Could you check a few things on this model? Use its own coordinates, in mm. Face numbers are marked on the shaded views. A direction names the side the tool comes from. Give positions to 0.01 mm unless a question says otherwise; leave off trailing zeros. Loops run counter-clockwise (first coordinate to the right, second up) from the corner with the lowest first, then second, coordinate; pieces in that order, holes last. Notation, with made-up numbers: M -1.75,-27.5 L 37.25,-27.5 A14 ccw 37.25,-18.5 Z; hole C 13.5,-6 d8. An arc over 180 degrees is marked long. Write each question's results on one line, items separated by ' | '. Start each with the question number.
from build123d import *

# Parameters (mm, degrees)
F0_W     = 101.5878766775
F0_H     = 24.442197755
F1_DEPTH = 20
F3_DEPTH = 25
F5_DEPTH = 25


with BuildPart() as f1:
    # F0 (on Top) → F1 (new body)
    with BuildSketch(Plane.XY):
        with Locations((0.3819093108, 12.2210988775)):
            Rectangle(F0_W, F0_H)
    extrude(amount=F1_DEPTH)

    # F2 (on face) → F3 (cut)
    with BuildSketch(Plane.XY.offset(20)):
        with BuildLine():
            ThreePointArc((-50.4120290279, 16.5795714258), (-49.5897410565, 20.6289075462), (-47.9984842241, 24.442197755))
            Line((-47.9984842241, 24.442197755), (-50.4120290279, 24.442197755))
            Line((-50.4120290279, 24.442197755), (-50.4120290279, 16.5795714258))
        make_face()
        with BuildLine():
            ThreePointArc((-47.9984842241, 0), (-49.6724374157, 4.6588518495), (-50.4120290279, 9.5537496105))
            Line((-50.4120290279, 9.5537496105), (-50.4120290279, 0))
            Line((-50.4120290279, 0), (-47.9984842241, 0))
        make_face()
        with BuildLine():
            Line((51.1758476496, 24.442197755), (47.9984171689, 24.442197755))
            ThreePointArc((47.9984171689, 24.442197755), (50.12222675, 20.4607446272), (51.1758476496, 16.0729867548))
            Line((51.1758476496, 16.0729867548), (51.1758476496, 24.442197755))
        make_face()
        with BuildLine():
            Line((51.1758476496, 0), (51.1758476496, 12.2210988775))
            ThreePointArc((51.1758476496, 12.2210988775), (50.425198292, 5.9349952856), (48.2219271362, 0))
            Line((48.2219271362, 0), (51.1758476496, 0))
        make_face()
    extrude(amount=-F3_DEPTH, mode=Mode.SUBTRACT)

    # F4 (on face) → F5 (cut)
    with BuildSketch(Plane.XY.offset(20)):
        with BuildLine():
            ThreePointArc((-47.9984842241, 24.442197755), (-45.641486399, 24.1705843884), (-43.4080474079, 23.3699828386))
            Line((-43.4080474079, 23.3699828386), (44.5075258613, 23.3699828386))
            ThreePointArc((44.5075258613, 23.3699828386), (46.1724950081, 24.1681037554), (47.9984171689, 24.442197755))
            Line((47.9984171689, 24.442197755), (-47.9984842241, 24.442197755))
        make_face()
    extrude(amount=-F5_DEPTH, mode=Mode.SUBTRACT)


solid = f1.part
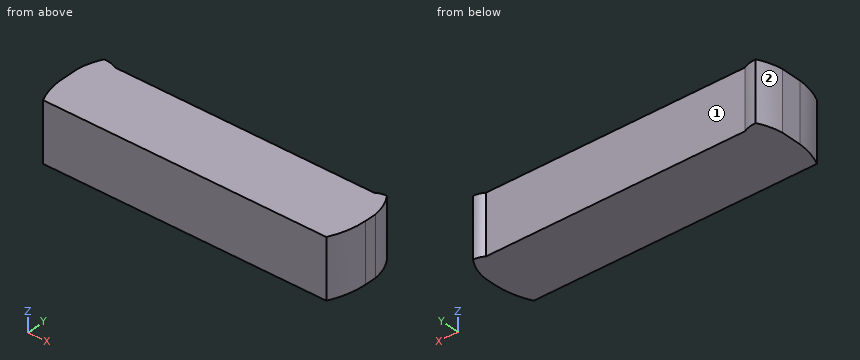
1) If we section it at A-A on z = 8.5: Write out the boundary of the cut face in (x, y), plus the area to 3 significant figures.
2) Which directions (+Z, -Z, +X, -X, +Y, -Y) give clear straight access to the entire face, cutting with the end or side of a thin tool? Please do the marked faces 1 and 2.
3) Please list where these lines run through material, in increasing order: line 1 (Y direction, x = -16.5, z = 8.5); line 2 (X direction, y = 12, z = 15.5); line 3 (X direction, y = 21.25, z = 5). Write a range as from..to.
4) If we section it at C-C on y = 4.25: Write out the boundary of the cut face in (x, z).
5) I'm going to push flat-ended pins straight in: P1, Ø8, axis at y = 4, z = 16, coming from the +X side; P2, Ø8, axis at y = 4, z = 12, coming from the -X side; P3, Ø10, axis at x = -11.5, z = 8.5, coming from the +Y side. Where does each tip first touch, or does it pass through?
6) If we section it at B-B on x = -24: Write out the boundary of the cut face in (y, z).
Calculated:
1) outline: M -50.41,9.55 A25.43 ccw -48,0 L 48.22,0 A26.82 ccw 51.18,12.22 L 51.18,16.07 A17.79 ccw 48,24.44 A6.22 ccw 44.51,23.37 L -43.41,23.37 A10.36 ccw -48,24.44 A21.23 ccw -50.41,16.58 Z | area: 2,350 mm2
2) face 1: +Z, -Z, +Y | face 2: +Z, -Z, -X, +Y
3) line 1: y = 0..23.37 | line 2: x = -50.41..51.17 | line 3: x = -49.39..49.8
4) outline: M -49.57,0 L 49.96,0 L 49.96,20 L -49.57,20 Z
5) P1: stops at x = 50.84 | P2: stops at x = -50.28 | P3: stops at y = 23.37
6) outline: M 0,0 L 23.37,0 L 23.37,20 L 0,20 Z
